Build history of the part. All positions in model axes, mm. A direction names the side the tool comes from. Coordinates: 2 decimals unless noted, no trailing zeros. Loops run counter-clockwise (first coordinate to the right, second up) from the corner with the lowest first, then second, coordinate; pieces in that order, holes last.
(1) Wall check: L1, parallel to X at y = 9.5, z = 15; L2, parallel to X at y = -0.5, z = 3.75 (3 decimals); L3, parallel to Y at x = 32, z = 2.5. Give the ranges that are in metal, low to high.
(2) Slice it at C-C (y = 2.5). Give the cut face in (x, z) (3 decimals).
(3) Tool access for faces 5 (the face through (8, 0, 6.35)), 6 (the face through (12.77, 9.523, 3.219)), 7 (the face through (29, 0, 6)): list every direction of +Z, -Z, +X, -X, +Y, -Y with a clear straight run to the whole face (end or side of a thin tool).
(4) Slice it at D-D (x = 36.5). Give the cut face in (y, z), and give its area (3 significant figures).
(5) Slice it at B-B (x = 12.7). Give the cut face in (y, z) (3 decimals).
(6) Slice it at A-A (z = 17.75). Give the cut face in (x, y), and give its area (3 significant figures).
(7) Flat gauge pins, fed straight in: P1, Ø3, axis at x = 22, y = 0.5, coming from the +Z side; P2, Ø1, axis at x = 24.5, z = 10.5, coming from the -Y side; P3, Ø3, axis at x = 4, y = -10, coming from the +Z side. Where does each tip first touch, or does it go through?
(8) Two-plate mould, pull along X, no slides. Class faces 1 (the face through (6.35, 7, 12)), 2 (the face through (19, 3, 0)), 3 (the face through (9.525, 0, 3)), 4 (the face through (38.1, 6, 10)): pulls with the +X half, pulls with the -X half, needs draft (parallel to the pull), parting line crosses it, or undercut.
from build123d import *

# Parameters (mm, degrees)
F0_W      = 6.35
F0_H      = 25.4
F1_DEPTH  = 12.7
F2_W      = 12.7
F2_H      = 6.35
F3_DEPTH  = 25.4
F4_W      = 19.05
F4_H      = 12.7
F5_DEPTH  = 12.7
F7_DEPTH  = 19.05
F9_DEPTH  = 6.35
F10_W     = 6.35
F10_H     = 12.698938
F11_DEPTH = 25.4


with BuildPart() as f1:
    # F0 (on Front) → F1 (new body, symmetric)
    with BuildSketch(Plane.XZ):
        with Locations((3.175, 12.7)):
            Rectangle(F0_W, F0_H)
    extrude(amount=F1_DEPTH, both=True)

    # F2 (on face) → F3 (join)
    with BuildSketch(Plane.XZ.offset(12.7)):
        with Locations((12.7, 3.175)):
            Rectangle(F2_W, F2_H)
    extrude(amount=-F3_DEPTH)

    # F4 (on face) → F5 (join)
    with BuildSketch(Plane(origin=(0, 12.7, 0), x_dir=(-1, 0, 0), z_dir=(0, 1, 0))):
        with Locations((-28.575, 6.35)):
            Rectangle(F4_W, F4_H)
    extrude(amount=-F5_DEPTH)

    # F6 (on face) → F7 (join)
    with BuildSketch(Plane.YZ.offset(38.1)):
        Polygon((0, 12.7), (12.7, 12.7), (12.7, 25.4), align=None)
    extrude(amount=-F7_DEPTH)

    # F8 (on face) → F9 (cut)
    with BuildSketch(Plane(origin=(0, 0, 0), x_dir=(0, -1, 0), z_dir=(-1, 0, 0))):
        Polygon((-12.7, 25.4), (12.7, 0), (12.7, 25.4), align=None)
    extrude(amount=-F9_DEPTH, mode=Mode.SUBTRACT)

    # F10 (on face) → F11 (cut)
    with BuildSketch(Plane.XY.offset(6.35)):
        with Locations((12.7, -0.000531)):
            Rectangle(F10_W, F10_H)
        with BuildLine():
            ThreePointArc((15.875, 6.348938), (12.7, 9.523938), (9.525, 6.348938))
            Line((9.525, 6.348938), (15.875, 6.348938))
        make_face()
        with BuildLine():
            Line((15.875, -6.35), (9.525, -6.35))
            ThreePointArc((9.525, -6.35), (12.7, -9.525), (15.875, -6.35))
        make_face()
    extrude(amount=-F11_DEPTH, mode=Mode.SUBTRACT)


solid = f1.part
Response values:
1. L1: x = 0 to 6.35, 19.05 to 38.1
1. L2: x = 0 to 9.525, 15.875 to 19.05
1. L3: y = 0 to 12.7
2. outline: (0, 0) - (9.525, 0) - (9.525, 6.35) - (6.35, 6.35) - (6.35, 15.2) - (0, 15.2) - close; (15.875, 0) - (38.1, 0) - (38.1, 15.2) - (19.05, 15.2) - (19.05, 6.35) - (15.875, 6.35) - close
3. face 5: +Z, +Y, -Y
3. face 6: +Z, -Z
3. face 7: +Z, -Z, +X, -Y
4. outline: (0, 0) - (12.7, 0) - (12.7, 25.4) - (0, 12.7) - close
4. area: 242 mm2
5. outline: (-12.7, 0) - (-9.525, 0) - (-9.525, 6.35) - (-12.7, 6.35) - close; (9.524, 0) - (12.7, 0) - (12.7, 6.35) - (9.524, 6.35) - close
6. outline: (0, 5.05) - (6.35, 5.05) - (6.35, 12.7) - (0, 12.7) - close; (19.05, 5.05) - (38.1, 5.05) - (38.1, 12.7) - (19.05, 12.7) - close
6. area: 194 mm2
7. P1: stops at z = 14.7
7. P2: stops at y = 0
7. P3: stops at z = 4.2
8. face 1: undercut
8. face 2: needs draft
8. face 3: undercut
8. face 4: pulls with the +X half
